```python
from build123d import *

# Parameters (mm, degrees)
CROQUIS1_R     = 5
EXTRUIR1_DEPTH = 2
VACIADO1_T     = -1
CROQUIS2_R     = 4
EXTRUIR2_DEPTH = 10
CROQUIS4_R     = 2
EXTRUIR4_DEPTH = 3


with BuildPart() as part:
    # Croquis1 → Extruir1 (new body)
    with BuildSketch(Plane.XY):
        Circle(CROQUIS1_R)
    extrude(amount=EXTRUIR1_DEPTH)

    # Vaciado1
    vaciado1_openings = [part.faces().sort_by_distance(p)[0] for p in [
        (0, 0, 2),
    ]]
    offset(amount=VACIADO1_T, openings=vaciado1_openings, kind=Kind.INTERSECTION)

    # Croquis2 → Extruir2 (add)
    with BuildSketch(Plane(origin=(0, 0, 0), x_dir=(-1, 0, 0), z_dir=(0, 0, -1))):
        with Locations(Location((0, 0, 0), (0, 0, 180))):  # turned: the seam where the file's is
            Circle(CROQUIS2_R)
    extrude(amount=EXTRUIR2_DEPTH)

    # Simetría3: part across plane


with BuildPart() as part_1:
    add(part.part)
    add(part.part.mirror(Plane(origin=(0, 0, -10), x_dir=(1, 0, 0), z_dir=(0, 0, -1))))

    # Croquis4 → Extruir4 (add)
    with BuildSketch(Plane.XY.offset(1)):
        Circle(CROQUIS4_R)
    extrude(amount=EXTRUIR4_DEPTH)


solid = part_1.part
```
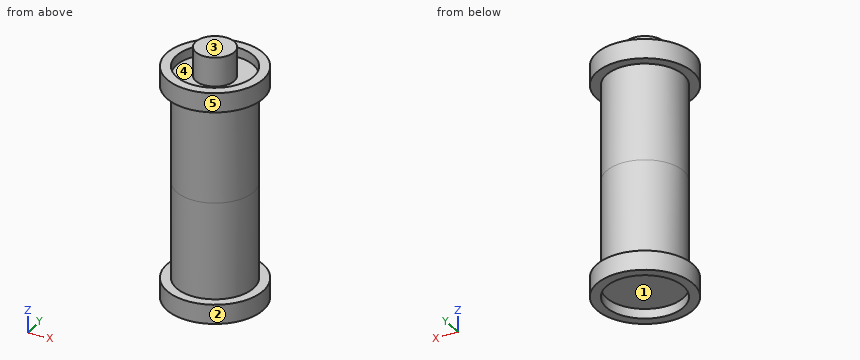
The model under review builds one solid part; all positions refer to its coordinate system, in mm. Face numbers are marked on the shaded views. A direction names the side the tool comes from. Coordinates: 2 decimals unless noted, no trailing zeros. Order: outer loops, then holes, each group sorted by start corner. A loop starts at its lowest first (then second) coordinate and runs counter-clockwise, first axis right, second up. Notation, with made-up numbers: M 30,89.5 L 73,89.5 A32 cw 73,120.5 Z; hole C 9.5,59.5 d9. An arc over 180 degrees is marked long. One line per question, with ' | ' between items.
(1) Machinability: for the marked faces 4 and 5, which of the approach directions +Z, -Z, +X, -X, +Y, -Y give a long, thin tool a straight path to every point of the face, cutting with its end or side? Answer none if there is none.
Geometry results:
face 4: +Z | face 5: +Z, -Z
(2) Add section A-A, the plane y = 4.75. Write out the cut boundary in (x, z), then the cut area to 3 significant figures.
Geometry results:
outline: M -1.56,-22 L 1.56,-22 L 1.56,-20 L -1.56,-20 Z; M -1.56,0 L 1.56,0 L 1.56,2 L -1.56,2 Z | area: 12.5 mm²
(3) The part is to be moulded in two halves that separate along X. For the marked faces 1, 2 and 3, say which applies: +X half, -X half, draft (parallel to the pull), parting line (faces both ways), or undercut.
Geometry results:
face 1: undercut | face 2: parting line | face 3: draft
(4) Insertion check: pin 1 (1 mm diameter, centred on x = -3.5, y = 2, fed in from +Z); pin 2 (1 mm diameter, centred on x = 1.5, z = -2, fed in from -Y); pin 3 (1 mm diameter, centred on y = -2, z = -14.5, fed in from +X). Each pin has a flat end and moves straight along its axis. Give the tip position at first contact, or say it passes through.
Geometry results:
pin 1: stops at z = 2 | pin 2: stops at y = -3.87 | pin 3: stops at x = 3.71
(5) Add section B-B, the plane x = 0. Write out the cut boundary in (y, z).
Geometry results:
outline: M -5,-22 L -4,-22 L -4,-21 L 4,-21 L 4,-22 L 5,-22 L 5,-20 L 4,-20 L 4,0 L 5,0 L 5,2 L 4,2 L 4,1 L 2,1 L 2,4 L -2,4 L -2,1 L -4,1 L -4,2 L -5,2 L -5,0 L -4,0 L -4,-20 L -5,-20 Z
(6) For probe 1 along Y at (x, z) = (0, 1.7); probe 2 along Z at (x, y) = (-3.5, -2); probe 3 along Y at (x, z) = (0, -21.4), list the stretches that pass through material, from the lowest coordinate up. Write a range as from..to.
Geometry results:
probe 1: y = -5..-4, -2..2, 4..5 | probe 2: z = -22..-20, 0..2 | probe 3: y = -5..-4, 4..5
(7) Add section D-D, the plane z = -2.25. Write out the cut boundary in (x, y).
Geometry results:
outline: C 0,0 d8
